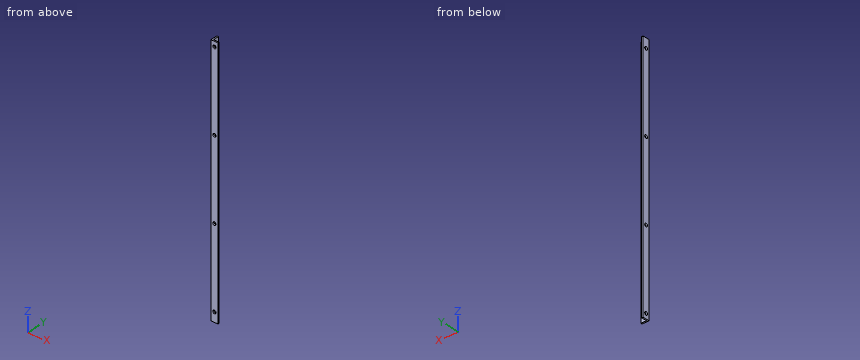
from build123d import *

# Parameters (mm, degrees)
EXTRUDE_1_DEPTH     = 350
SKETCH_2_R          = 2.25
CUT_EXTRUDE_1_DEPTH = 11
CUT_EXTRUDE_2_REACH = 12
SKETCH_3_R          = 2.25


with BuildPart() as part:
    # Эскиз1 → Бобышка-Вытянуть1 (new body)
    with BuildSketch(Plane.XY):
        Polygon((0, 0), (0, 10), (2, 10), (2, 2), (10, 2), (10, 0), align=None)
    extrude(amount=EXTRUDE_1_DEPTH)

    # Эскиз2 → Вырез-Вытянуть1 (cut, through all)
    with BuildSketch(Plane.ZY):
        with Locations((7, 5)):
            Circle(SKETCH_2_R)
        with Locations((117, 5)):
            Circle(SKETCH_2_R)
        with Locations((227, 5)):
            Circle(SKETCH_2_R)
        with Locations((337, 5)):
            Circle(SKETCH_2_R)
    extrude(amount=-CUT_EXTRUDE_1_DEPTH, mode=Mode.SUBTRACT)

    # Эскиз3 → Вырез-Вытянуть2 (cut, up to next)
    with BuildSketch(Plane.XZ, mode=Mode.PRIVATE) as cut_extrude_2_sk1:
        with Locations((5, 343)):
            Circle(SKETCH_3_R)
    cut_extrude_2_tool1 = extrude(cut_extrude_2_sk1.sketch, amount=-CUT_EXTRUDE_2_REACH, mode=Mode.PRIVATE) & part.part
    add(cut_extrude_2_tool1.solids().sort_by_distance((5, 0, 343))[0], mode=Mode.SUBTRACT)
    # Эскиз3 → Вырез-Вытянуть2 (cut, up to next)
    with BuildSketch(Plane.XZ, mode=Mode.PRIVATE) as cut_extrude_2_sk2:
        with Locations((5, 233)):
            Circle(SKETCH_3_R)
    cut_extrude_2_tool2 = extrude(cut_extrude_2_sk2.sketch, amount=-CUT_EXTRUDE_2_REACH, mode=Mode.PRIVATE) & part.part
    add(cut_extrude_2_tool2.solids().sort_by_distance((5, 0, 233))[0], mode=Mode.SUBTRACT)
    # Эскиз3 → Вырез-Вытянуть2 (cut, up to next)
    with BuildSketch(Plane.XZ, mode=Mode.PRIVATE) as cut_extrude_2_sk3:
        with Locations((5, 123)):
            Circle(SKETCH_3_R)
    cut_extrude_2_tool3 = extrude(cut_extrude_2_sk3.sketch, amount=-CUT_EXTRUDE_2_REACH, mode=Mode.PRIVATE) & part.part
    add(cut_extrude_2_tool3.solids().sort_by_distance((5, 0, 123))[0], mode=Mode.SUBTRACT)
    # Эскиз3 → Вырез-Вытянуть2 (cut, up to next)
    with BuildSketch(Plane.XZ, mode=Mode.PRIVATE) as cut_extrude_2_sk4:
        with Locations((5, 13)):
            Circle(SKETCH_3_R)
    cut_extrude_2_tool4 = extrude(cut_extrude_2_sk4.sketch, amount=-CUT_EXTRUDE_2_REACH, mode=Mode.PRIVATE) & part.part
    add(cut_extrude_2_tool4.solids().sort_by_distance((5, 0, 13))[0], mode=Mode.SUBTRACT)


solid = part.part
The model under review builds one solid part; all positions refer to its coordinate system, in mm. Round coordinates to 2 decimals unless told otherwise and drop trailing zeros. Loops run counter-clockwise (first coordinate to the right, second up) from the corner with the lowest first, then second, coordinate; pieces in that order, holes last. Notation, with made-up numbers: (12.25, 61) - (36.25, 61) arc R29 ccw to (36.25, 84) - close; hole circle Ø7 at (78, 45.25). An arc over 180 degrees is marked (long way). Use CSV: the item, a comma, the result in double quotes.
(1) Take a section at A-A, the plane y = 5. Give the boundary of the cut face in (x, z).
Working result:
outline,"(0, 0) - (2, 0) - (2, 4.75) - (0, 4.75) - close; (0, 9.25) - (2, 9.25) - (2, 114.75) - (0, 114.75) - close; (0, 119.25) - (2, 119.25) - (2, 224.75) - (0, 224.75) - close; (0, 229.25) - (2, 229.25) - (2, 334.75) - (0, 334.75) - close; (0, 339.25) - (2, 339.25) - (2, 350) - (0, 350) - close"
(2) For line 1 (Z direction, x = 5, y = 1.15); line 2 (Y direction, x = 0.4, z = 227); line 3 (Z direction, x = 1, y = 4), list the stretches that pass through material, from the lowest coordinate up.
Working result:
line 1,"z = 0 to 10.75, 15.25 to 120.75, 125.25 to 230.75, 235.25 to 340.75, 345.25 to 350"
line 2,"y = 0 to 2.75, 7.25 to 10"
line 3,"z = 0 to 4.98, 9.02 to 114.98, 119.02 to 224.98, 229.02 to 334.98, 339.02 to 350"
(3) Take a section at B-B, the plane z = 317.5. Give the boundary of the cut face in (x, y).
Working result:
outline,"(0, 0) - (10, 0) - (10, 2) - (2, 2) - (2, 10) - (0, 10) - close"
(4) Clearance check with flat-ended pins moving along their axes: P1, Ø4, axis at y = 5, z = 227, coming from the +X side; P2, Ø5, axis at x = 5, z = 13, coming from the +Y side; P3, Ø5, axis at y = 5, z = 117, coming from the +X side. State where each tip first meets the part, or that it passes through.
Working result:
P1,"passes through"
P2,"stops at y = 2"
P3,"stops at x = 2"
